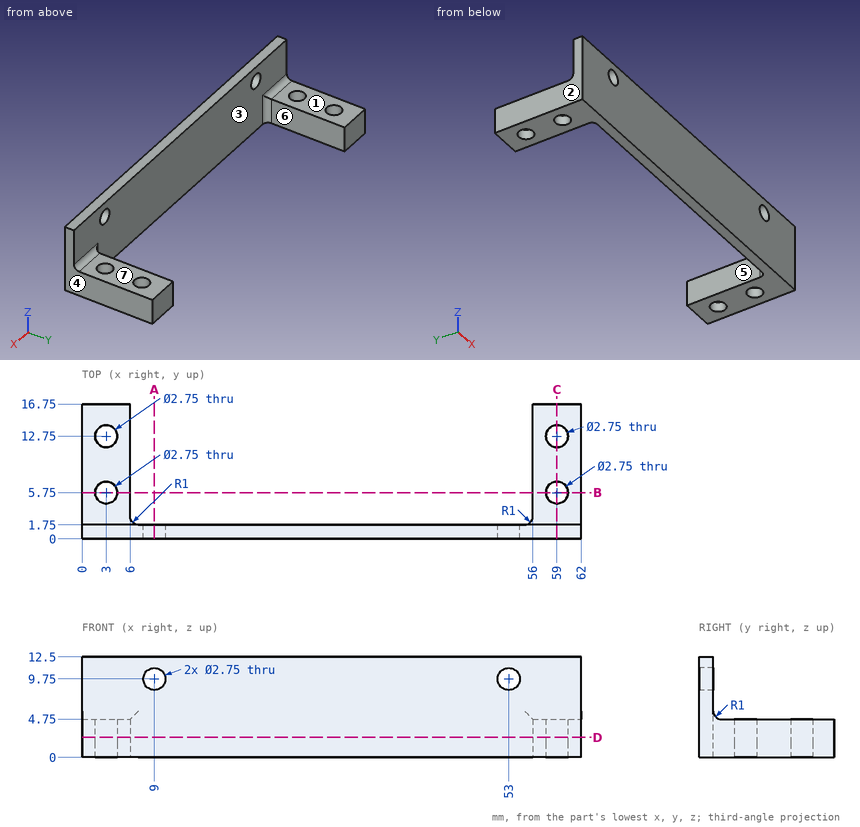
Part print with two shaded views. Sizes in mm from the minimum x, y, z corner. A direction names the side the tool comes from. Round coordinates to 2 decimals unless told otherwise and drop trailing zeros. Order: outer loops, then holes, each group sorted by start corner. A loop starts at its lowest first (then second) coordinate and runs counter-clockwise, first axis right, second up. Notation, with made-up numbers: (15.5, 70) - (65.5, 70) arc R30 ccw to (65.5, 103) - close; hole circle Ø9 at (-38, 29). An arc over 180 degrees is marked (long way). Answer in a Markdown table with one row per item. Add a question column.
(1) 3-axis set-ups, long thin cutter, end or side, ignore diameter. For the marked faces 1, 2 and 3: which of +Z, -Z, +X, -X, +Y, -Y reach the whole face in a straight line?
(2) Drop flat-ended pins along their axis: pin 1 Ø4 at (x, z) = (42.5, 5) entering from +Y; pin 2 Ø5 at (x, y) = (11, 6.5) entering from -Z; pin 3 Ø3 at (x, y) = (3, 10) entering from +Z. Give the stop position or say it passes through.
(3) Band-saw the part on A-A on x = 9. List the corners of the cut face in (y, z) (3 decimals), and give its area (3 significant figures).
(4) Band-saw the part on D-D on z = 2.5. List the corners of the cut face in (x, y) (3 decimals), and give its area (3 significant figures).
(5) Band-saw the part on C-C on x = 59. List the corners of the cut face in (y, z) (3 decimals), and give its area (3 significant figures).
(6) Mould opens along X. For the marked faces 4, 5, 6 and 7 say: +X half, -X half, draft (parallel to the pull), parting line (faces both ways), or undercut.
(7) Band-saw the part on B-B on y = 5.75. List the corners of the cut face in (x, z) (3 decimals).
(8) Probe L1, parallel to Y at x = 59, z = 2.8 (3 decimals); L2, parallel to X at y = 15.75, z = 2.5; L3, parallel to X at y = 0.9, z = 9.75 (3 decimals). List the from-to ranges inside material, lowest first. Write a range as [from, to].
Data:
| question | item | result |
|---|---|---|
| 1 | face 1 | +Z, +X, -X, +Y |
| 1 | face 2 | +Z, -Z, -X, +Y, -Y |
| 1 | face 3 | +Z, +Y |
| 2 | pin 1 | stops at y = 1.75 |
| 2 | pin 2 | passes through |
| 2 | pin 3 | stops at z = 4.75 |
| 3 | outline | (0, 0) - (1.75, 0) - (1.75, 8.375) - (0, 8.375) - close; (0, 11.125) - (1.75, 11.125) - (1.75, 12.5) - (0, 12.5) - close |
| 3 | area | 17.1 mm^2 |
| 4 | outline | (0, 0) - (62, 0) - (62, 16.75) - (56, 16.75) - (56, 2.75) arc R1 cw to (55, 1.75) - (7, 1.75) arc R1 cw to (6, 2.75) - (6, 16.75) - (0, 16.75) - close; hole circle Ø2.75 at (3, 5.75); hole circle Ø2.75 at (3, 12.75); hole circle Ø2.75 at (59, 5.75); hole circle Ø2.75 at (59, 12.75) |
| 4 | area | 265 mm^2 |
| 5 | outline | (0, 0) - (4.375, 0) - (4.375, 4.75) - (2.75, 4.75) arc R1 cw to (1.75, 5.75) - (1.75, 12.5) - (0, 12.5) - close; (7.125, 0) - (11.375, 0) - (11.375, 4.75) - (7.125, 4.75) - close; (14.125, 0) - (16.75, 0) - (16.75, 4.75) - (14.125, 4.75) - close |
| 5 | area | 67.2 mm^2 |
| 6 | face 4 | +X half |
| 6 | face 5 | undercut |
| 6 | face 6 | undercut |
| 6 | face 7 | draft |
| 7 | outline | (0, 0) - (1.625, 0) - (1.625, 4.75) - (0, 4.75) - close; (4.375, 0) - (6, 0) - (6, 4.75) - (4.375, 4.75) - close; (56, 0) - (57.625, 0) - (57.625, 4.75) - (56, 4.75) - close; (60.375, 0) - (62, 0) - (62, 4.75) - (60.375, 4.75) - close |
| 8 | L1 | y = [0, 4.375], [7.125, 11.375], [14.125, 16.75] |
| 8 | L2 | x = [0, 6], [56, 62] |
| 8 | L3 | x = [0, 7.625], [10.375, 51.625], [54.375, 62] |
